Design review of the part built by this model. Coordinates are the model's own, in mm. A direction names the side the tool comes from. Give positions to 0.01 mm unless a question says otherwise; leave off trailing zeros. Loops run counter-clockwise (first coordinate to the right, second up) from the corner with the lowest first, then second, coordinate; pieces in that order, holes last. Notation, with made-up numbers: (75.25, -5) -> (130.25, -5) arc R16 ccw to (130.25, 23) -> close; hole circle Ø6 at (-38, 8). An arc over 180 degrees is marked (long way). Use a Markdown table: item, result. Add a question column.
1. For faces 4 (the flat face through (-22, -10, 41)), 5 (the flat face through (-10, -10, 3)), 6 (the flat face through (0, -10, 24)), list the 3-axis set-ups (+Z, -Z, +X, -X, +Y, -Y) from which the entire face can be reached by the end or side of a thin tool; tool diameter is ignored.
2. Add section B-B (x = -16). State the section outline as (y, z) points, and give its area (3 significant figures).
3. To check wall thickness, follow line 1 (Z direction, x = 7.5, y = -2.25); line 2 (Z direction, x = -28.5, y = -10.5); line 3 (X direction, y = -12.5, z = 10.5). State the ranges of each line that lie inside material, in increasing order.
4. For pin 1 Ø3 at (y, z) = (-12.5, 24.5) entering from +X; pin 2 Ø6 at (x, y) = (12.5, -11.5) entering from +Z, all flat-tipped, find the tip position at first contact; note any pin that passes through.
5. Add section D-D (y = -1.25). State the section outline as (x, z) points, and give its area (3 significant figures).
6. Add section C-C (y = -9.5). State the section outline as (x, z) points, and give its area (3 significant figures).
7. Add section A-A (z = 27). State the section outline as (x, y) points.
8. Draft analysis for pull direction Z (two halves, no side actions). For faces 1 (the flat face through (8.6, -7.6, 5.5)), 2 (the cylindrical face through (11.602, -6.275, 1.479)), 3 (the flat face through (-42, -10, 22)), state which applies: pulls with the +Z half, pulls with the -Z half, needs draft (parallel to the pull), parting line crosses it, or undercut.
```python
from build123d import *

# Parameters (mm, degrees)
F1_DEPTH = 20
F2_R     = 1
F3_R     = 4
F4_DEPTH = 23.2


with BuildPart() as f1:
    # F0 (on Front) → F1 (new body)
    with BuildSketch(Plane.XZ):
        Polygon((-44, 0), (20.290818, 0), (20.290818, 3), (-2, 3), (-42, 3), (-42, 41), (-2, 41), (-2, 3.422746), (20.290818, 3.5), (20.290818, 5.5), (0, 5.5), (0, 44), (-44, 44), align=None)
    extrude(amount=F1_DEPTH)

    # F2
    f2_edges = [f1.edges().sort_by_distance(p)[0] for p in [
        (-2, -10, 41),
        (-42, -10, 41),
        (-42, -10, 3),
        (0, -10, 5.5),
        (0, -10, 44),
        (-44, -10, 44),
        (-44, -10, 0),
        (-2, -10, 3.422746),
    ]]
    fillet(f2_edges, radius=F2_R)

    # F3 (on Top) → F4 (cut)
    with BuildSketch(Plane.XY):
        with Locations((12.122351, -10.240848)):
            Circle(F3_R)
    extrude(amount=F4_DEPTH, mode=Mode.SUBTRACT)


solid = f1.part
```
Taken from the geometry:
| question | item | result |
|---|---|---|
| 1 | face 4 | +Y, -Y |
| 1 | face 5 | +X, +Y, -Y |
| 1 | face 6 | +Z, +X, +Y, -Y |
| 2 | outline | (-20, 0) -> (0, 0) -> (0, 3) -> (-20, 3) -> close; (-20, 41) -> (0, 41) -> (0, 44) -> (-20, 44) -> close |
| 2 | area | 120 mm^2 |
| 3 | line 1 | z = 0 to 3, 3.46 to 5.5 |
| 3 | line 2 | z = 0 to 3, 41 to 44 |
| 3 | line 3 | x = -44 to -42, -2 to 0 |
| 4 | pin 1 | stops at x = 0 |
| 4 | pin 2 | stops at z = 5.5 |
| 5 | outline | (-44, 1) arc R1 ccw to (-43, 0) -> (20.29, 0) -> (20.29, 3) -> (-41, 3) arc R1 cw to (-42, 4) -> (-42, 40) arc R1 cw to (-41, 41) -> (-3, 41) arc R1 cw to (-2, 40) -> (-2, 4.43) arc R1 ccw to (-1, 3.43) -> (20.29, 3.5) -> (20.29, 5.5) -> (1, 5.5) arc R1 cw to (0, 6.5) -> (0, 43) arc R1 ccw to (-1, 44) -> (-43, 44) arc R1 ccw to (-44, 43) -> close |
| 5 | area | 517 mm^2 |
| 6 | outline | (-44, 1) arc R1 ccw to (-43, 0) -> (8.19, 0) -> (8.19, 3) -> (-41, 3) arc R1 cw to (-42, 4) -> (-42, 40) arc R1 cw to (-41, 41) -> (-3, 41) arc R1 cw to (-2, 40) -> (-2, 4.43) arc R1 ccw to (-1, 3.43) -> (8.19, 3.46) -> (8.19, 5.5) -> (1, 5.5) arc R1 cw to (0, 6.5) -> (0, 43) arc R1 ccw to (-1, 44) -> (-43, 44) arc R1 ccw to (-44, 43) -> close; (16.05, 0) -> (20.29, 0) -> (20.29, 3) -> (16.05, 3) -> close; (16.05, 3.49) -> (20.29, 3.5) -> (20.29, 5.5) -> (16.05, 5.5) -> close |
| 6 | area | 478 mm^2 |
| 7 | outline | (-44, -20) -> (-42, -20) -> (-42, 0) -> (-44, 0) -> close; (-2, -20) -> (0, -20) -> (0, 0) -> (-2, 0) -> close |
| 8 | face 1 | pulls with the +Z half |
| 8 | face 2 | needs draft |
| 8 | face 3 | undercut |
